For this review, take the finished solid that the model builds, in its own axes (mm). Face numbers are marked on the shaded views. Give positions to 0.01 mm unless a question says otherwise; leave off trailing zeros. Write each loop counter-clockwise with the first axis right and the second up, starting at its lowest first coordinate (ties: lowest second). Pieces come first, ordered by that corner, then holes. Notation, with made-up numbers: M 7,4 L 42,4 A29 cw 42,31 Z; hole C -31,47.5 d4. An arc over 180 degrees is marked long. One line per item, written item: value. Start each with the question number.
Item 1: Clearance check with flat-ended pins moving along their axes: pin 1 Ø4 at (x, z) = (5.5, 34.5) entering from -Y; pin 2 Ø11 at (x, y) = (-1.5, 12.5) entering from -Z; pin 3 Ø10 at (x, y) = (-36, -15) entering from -Z; pin 4 Ø3 at (x, z) = (5.5, 28) entering from +Y. State where each tip first meets the part, or that it passes through.
Item 2: Consider section B-B, the plane z = 26.5. Write out the cut boundary in (x, y), and give its area (3 significant figures).
Item 3: Consider section A-A, the plane x = 0. Write out the cut boundary in (y, z), and give its area (3 significant figures).
Item 4: Mouldability with a two-part tool opening along Y and no side actions: class the marked faces 1 and 2 as released by +Y, released by -Y, zero draft, split by the parting line, or undercut.
Item 5: Consider section C-C, the plane z = 38. Write out the cut boundary in (x, y).
Item 6: To check wall thickness, follow probe 1 along X at (y, z) = (39.5, 27); probe 2 along Y at (x, z) = (-4, 23); probe 3 along Y at (x, z) = (-52.5, 44.5). State the ranges of each line that lie inside material, in increasing order.
```python
from build123d import *

# Parameters (mm, degrees)
F3_R     = 11.001579
F4_DEPTH = 25.4


with BuildPart() as f1:
    # F0 (on Right) → F1 (revolve)
    with BuildSketch(Plane.YZ):
        Polygon((-56.302847, 48.771877), (0, 0), (0, -25.4), (12.7, -25.4), (12.7, 0), (2.291456, 0), (-54.740725, 50.534844), align=None)
    revolve(axis=Axis((0, 12.7, -12.7), (0, 0, 1)))

    # F3 (on face) → F4 (cut)
    with BuildSketch(Plane(origin=(0, 0, -25.4), x_dir=(1, 0, 0), z_dir=(0, 0, -1))):
        with Locations((0, -12.841756)):
            Circle(F3_R)
    extrude(amount=-F4_DEPTH, mode=Mode.SUBTRACT)


solid = f1.part
```
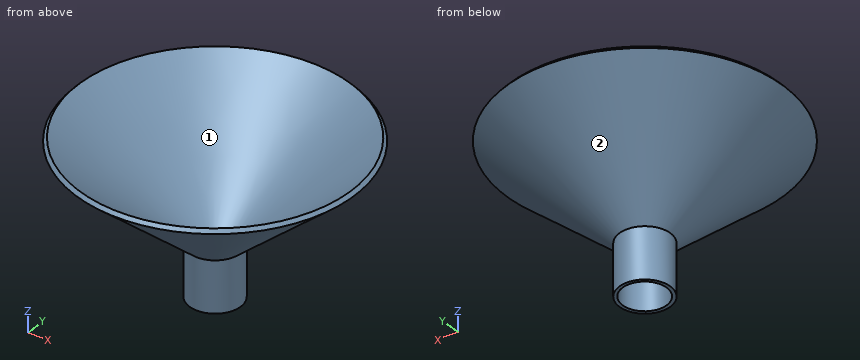
Model answer:
1. pin 1: stops at y = -41.87
1. pin 2: passes through
1. pin 3: stops at z = 24.02
1. pin 4: stops at y = 59.14
2. outline: C 0,12.7 d86.58; hole C 0,12.7 d80.63
2. area: 782 mm2
3. outline: M -56.3,48.77 L 0,0 L 0,-25.4 L 1.84,-25.4 L 1.84,0 L 2.29,0 L -54.74,50.53 Z; M 23.11,0 L 23.84,0 L 23.84,-25.4 L 25.4,-25.4 L 25.4,0 L 81.7,48.77 L 80.14,50.53 Z
3. area: 378 mm2
4. face 1: undercut
4. face 2: split by the parting line
5. outline: C 0,12.7 d113.14; hole C 0,12.7 d106.59
6. probe 1: x = -34.73 to -30.87, 30.87 to 34.73
6. probe 2: y = -26.35 to -23.45, 48.85 to 51.75
6. probe 3: y = -24.03 to -17.63, 43.03 to 49.43
